Verification items for the finished model (mm, model axes). Face numbers are marked on the shaded views. Coordinates: 2 decimals unless noted, no trailing zeros. Loops run counter-clockwise (first coordinate to the right, second up) from the corner with the lowest first, then second, coordinate; pieces in that order, holes last.
Q1. Sectioned sample at C-C (x = 30.5). Enter the section's corners in (y, z) (3 decimals), then the cut area to 3 significant figures.
Q2. Go/stop test with flat-tipped pins: P1, Ø4, axis at y = 10, z = 9, coming from the -X side; P2, Ø10, axis at x = 29.5, y = -8, coming from the +Z side; P3, Ø2, axis at x = 28, z = -9.5, coming from the +Y side. Record where each tip stops, or that it passes through.
Q3. Sectioned sample at B-B (z = 0). Count the separate pieces of the cut face and the enclosed holes in it, then the cut area to 3 significant figures.
Q4. Mould release check, pull along Y, two halves, no side actions. Record for the marked faces 1, 2 and 3: +Y half, -Y half, draft (parallel to the pull), parting line (faces both ways), or undercut.
Q5. Material ranges on probe 1 along Y at (x, z) = (8, -3.75); probe 2 along Y at (x, z) = (16.25, 0); probe 3 along Y at (x, z) = (13, 1), recorded low to high.
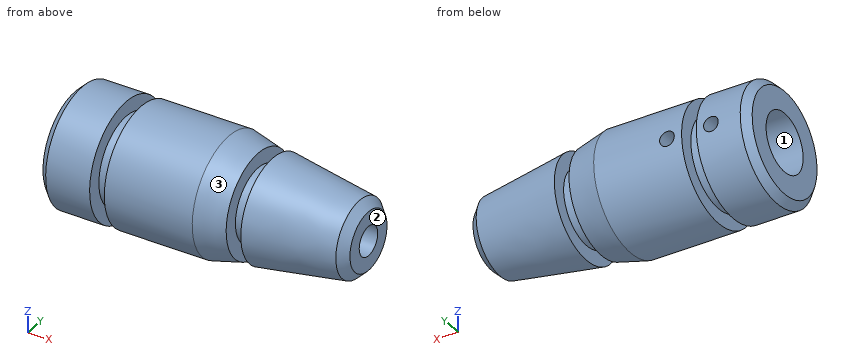
```python
from build123d import *
from OCP.BRepFilletAPI import BRepFilletAPI_MakeChamfer

# Parameters (mm, degrees)
CHAMFER1_SIZE           = 1.5875
CHAMFER1_SIZE2          = 1.898209315
CUT_EXTRUDE1_REACH      = 71.561
CUT_EXTRUDE1_END_RADIUS = 6.35
SKETCH2_R               = 1.5875


with BuildPart() as part:
    # Sketch1 → Revolve1 (revolve)
    with BuildSketch(Plane.XY, mode=Mode.PRIVATE) as revolve1_sk:
        Polygon((0, 6.35), (0, 12.7), (11.1125, 12.7), (11.1125, 9.525), (14.2875, 9.525), (14.2875, 12.7), (33.3375, 12.7), (39.6875, 11.1125), (39.6875, 7.9375), (42.8625, 7.9375), (42.8625, 11.1125), (63.5, 7.9375), (63.5, 3.175), (25.4, 3.175), (20.6375, 6.35), align=None)
    revolve(revolve1_sk.sketch.rotate(Axis((0, 0, 0), (1, 0, 0)), 90), axis=Axis((0, 0, 0), (1, 0, 0)))

    # Chamfer1: one chamfer whose edges measure the first distance from different faces: ONE call of the kernel's chamfer builder (chamfer() names one face for all edges)
    chamfer1_edges_1 = [part.edges().sort_by_distance(p)[0] for p in [
        (0, 0, -12.7),
    ]]
    chamfer1_edges_2 = [part.edges().sort_by_distance(p)[0] for p in [
        (63.5, 0, -7.9375),
    ]]
    chamfer1_side_2 = [part.faces().sort_by_distance(p)[0] for p in [
        (63.5, 0, -7.712993597),
    ]]
    chamfer1 = BRepFilletAPI_MakeChamfer(part.part.solid().wrapped)
    for e in chamfer1_edges_1:
        chamfer1.Add(CHAMFER1_SIZE, e.wrapped)
    for e in chamfer1_edges_2:
        chamfer1.Add(CHAMFER1_SIZE, CHAMFER1_SIZE2, e.wrapped, chamfer1_side_2[0].wrapped)  # the first distance lies on this face
    add(Compound.cast(chamfer1.Shape()), mode=Mode.REPLACE)

    # Cut-Extrude1: up to this cylinder (the profile starts outside it)
    cut_extrude1_end = Plane(origin=(12.7, 0, 0), z_dir=(-1, 0, 0)) * Cylinder(CUT_EXTRUDE1_END_RADIUS, 166.347, mode=Mode.PRIVATE)
    # Sketch2 → Cut-Extrude1 (cut, up to the surface)
    with BuildSketch(Plane(origin=(0, 12.7, 0), x_dir=(1, 0, 0), z_dir=(0, 1, 0)), mode=Mode.PRIVATE) as cut_extrude1_sk1:
        with Locations(Location((7.9375, 0, 0), (0, 0, 270))):
            Circle(SKETCH2_R)
    cut_extrude1_tool1 = extrude(cut_extrude1_sk1.sketch, amount=-CUT_EXTRUDE1_REACH, mode=Mode.PRIVATE) - cut_extrude1_end
    add(cut_extrude1_tool1.solids().sort_by_distance((7.9375, 12.7, 0))[0], mode=Mode.SUBTRACT)
    # Sketch2 → Cut-Extrude1 (cut, up to the surface)
    with BuildSketch(Plane(origin=(0, 12.7, 0), x_dir=(1, 0, 0), z_dir=(0, 1, 0)), mode=Mode.PRIVATE) as cut_extrude1_sk2:
        with Locations(Location((17.4625, 0, 0), (0, 0, 270))):
            Circle(SKETCH2_R)
    cut_extrude1_tool2 = extrude(cut_extrude1_sk2.sketch, amount=-CUT_EXTRUDE1_REACH, mode=Mode.PRIVATE) - cut_extrude1_end
    add(cut_extrude1_tool2.solids().sort_by_distance((17.4625, 12.7, 0))[0], mode=Mode.SUBTRACT)


solid = part.part
```
Geometry check:
1. outline: circle Ø25.4 at (0, 0); hole circle Ø6.35 at (0, 0)
1. area: 475 mm2
2. P1: stops at x = 0.34
2. P2: stops at z = 12.34
2. P3: stops at y = 9.44
3. separate pieces: 4
3. enclosed holes: 0
3. area: 826 mm2
4. face 1: undercut
4. face 2: draft
4. face 3: parting line
5. probe 1: y = -12.13 to -5.12, 5.12 to 12.13
5. probe 2: y = -12.7 to -6.35
5. probe 3: y = -9.47 to -6.27, 6.27 to 9.47
